```python
from build123d import *

# Parameters (mm, degrees)
EXTRUDE_1_DEPTH     = 6
SKETCH_2_R          = 1.35
CUT_EXTRUDE_1_DEPTH = 6
SKETCH_4_R          = 1.6
CUT_EXTRUDE_2_DEPTH = 6


with BuildPart() as part:
    # 草图1 → 凸台-拉伸1 (new body)
    with BuildSketch(Plane(origin=(0, 0, 0), x_dir=(1, 0, 0), z_dir=(0, 1, 0))):
        with BuildLine():
            Line((45, -30), (45, 30))
            Line((45, 30), (25, 30))
            Line((25, 30), (-1.65246447, 28.452053725))
            ThreePointArc((-1.65246447, 28.452053725), (-28.5, 0), (-1.65246447, -28.452053725))
            Line((-1.65246447, -28.452053725), (25, -30))
            Line((25, -30), (45, -30))
        make_face()
    extrude(amount=EXTRUDE_1_DEPTH)

    # 草图2 → 切除-拉伸1 (cut)
    with BuildSketch(Plane(origin=(0, 6, 0), x_dir=(1, 0, 0), z_dir=(0, 1, 0))):
        with Locations(Location((-13.435028843, 13.435028843, 0), (0, 0, 270))):
            Circle(SKETCH_2_R)
        with Locations(Location((13.435028843, 13.435028843, 0), (0, 0, 270))):
            Circle(SKETCH_2_R)
        with Locations(Location((13.435028843, -13.435028843, 0), (0, 0, 270))):
            Circle(SKETCH_2_R)
        with Locations(Location((-13.435028843, -13.435028843, 0), (0, 0, 270))):
            Circle(SKETCH_2_R)
    extrude(amount=-CUT_EXTRUDE_1_DEPTH, mode=Mode.SUBTRACT)

    # 草图4 → 切除-拉伸2 (cut)
    with BuildSketch(Plane(origin=(0, 6, 0), x_dir=(1, 0, 0), z_dir=(0, 1, 0))):
        with Locations(Location((35, 20, 0), (0, 0, 270))):
            Circle(SKETCH_4_R)
        with Locations(Location((35, 10, 0), (0, 0, 270))):
            Circle(SKETCH_4_R)
        with Locations(Location((35, -20, 0), (0, 0, 270))):
            Circle(SKETCH_4_R)
        with Locations(Location((35, -10, 0), (0, 0, 270))):
            Circle(SKETCH_4_R)
    extrude(amount=-CUT_EXTRUDE_2_DEPTH, mode=Mode.SUBTRACT)


solid = part.part
```
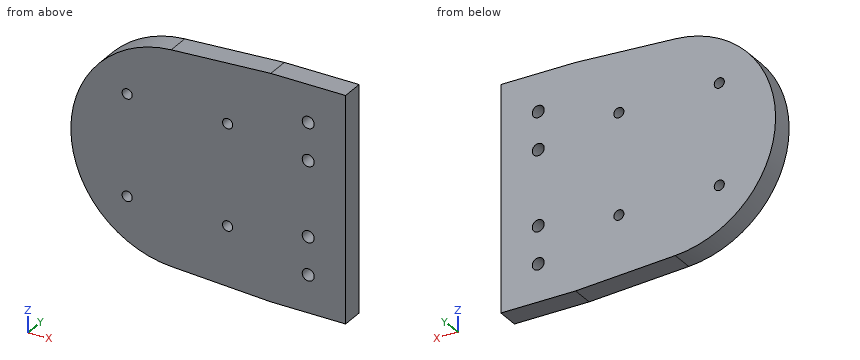
CAD build for the part. Positions are in the model's coordinates, mm. Round coordinates to 2 decimals unless told otherwise and drop trailing zeros. Order: outer loops, then holes, each group sorted by start corner. A loop starts at its lowest first (then second) coordinate and runs counter-clockwise, first axis right, second up.
Q1. Drop flat-ended pins along their axis: pin 1 (3.5 mm diameter, centred on x = 35, z = 10, fed in from +Y); pin 2 (2.5 mm diameter, centred on x = 13.44, z = -13.44, fed in from -Y); pin 3 (1 mm diameter, centred on x = -13, y = 5.5, fed in from +Z). Give the stop position or say it passes through.
Q2. Slice it at B-B (z = -20). Write the cut outline in (x, y).
Q3. Wall check: L1, parallel to Z at x = -13.5, y = 2.4; L2, parallel to X at y = 4.8, z = 12.5; L3, parallel to X at y = 3.9, z = 13.5. Give the ranges that are in metal, low to high.
Q4. Slice it at A-A (x = 35). Write the cut outline in (y, z), and give its area (3 significant figures).
Q5. Slice it at C-C (y = 2.4). State how many separate pieces and enclosed holes the cut face has, and give its area (3 significant figures).
Q6. Slice it at D-D (z = 10). Write the cut outline in (x, y).
Results below:
1. pin 1: stops at y = 6
1. pin 2: passes through
1. pin 3: stops at z = 25.61
2. outline: (-20.3, 0) - (33.4, 0) - (33.4, 6) - (-20.3, 6) - close; (36.6, 0) - (45, 0) - (45, 6) - (36.6, 6) - close
3. L1: z = -25.1 to -14.78, -12.09 to 12.09, 14.78 to 25.1
3. L2: x = -25.61 to -14.41, -12.46 to 12.46, 14.41 to 45
3. L3: x = -25.1 to -14.78, -12.09 to 12.09, 14.78 to 45
4. outline: (0, -30) - (6, -30) - (6, -21.6) - (0, -21.6) - close; (0, -18.4) - (6, -18.4) - (6, -11.6) - (0, -11.6) - close; (0, -8.4) - (6, -8.4) - (6, 8.4) - (0, 8.4) - close; (0, 11.6) - (6, 11.6) - (6, 18.4) - (0, 18.4) - close; (0, 21.6) - (6, 21.6) - (6, 30) - (0, 30) - close
4. area: 283 mm2
5. separate pieces: 1
5. enclosed holes: 8
5. area: 3,880 mm2
6. outline: (-26.69, 0) - (33.4, 0) - (33.4, 6) - (-26.69, 6) - close; (36.6, 0) - (45, 0) - (45, 6) - (36.6, 6) - close
